Geometry check sheet. Reference: drawing and pictorial views, mm from the part's lowest x, y, z. Coordinates: 2 decimals unless noted, no trailing zeros. Write each loop counter-clockwise with the first axis right and the second up, starting at its lowest first coordinate (ties: lowest second). Pieces come first, ordered by that corner, then holes. Notation, with made-up numbers: (85, 26.25) -> (118, 26.25) arc R10 ccw to (118, 36.25) -> close; hole circle Ø10 at (37, -30). An arc over 180 degrees is marked (long way). Answer in a Markdown table with one row per item.
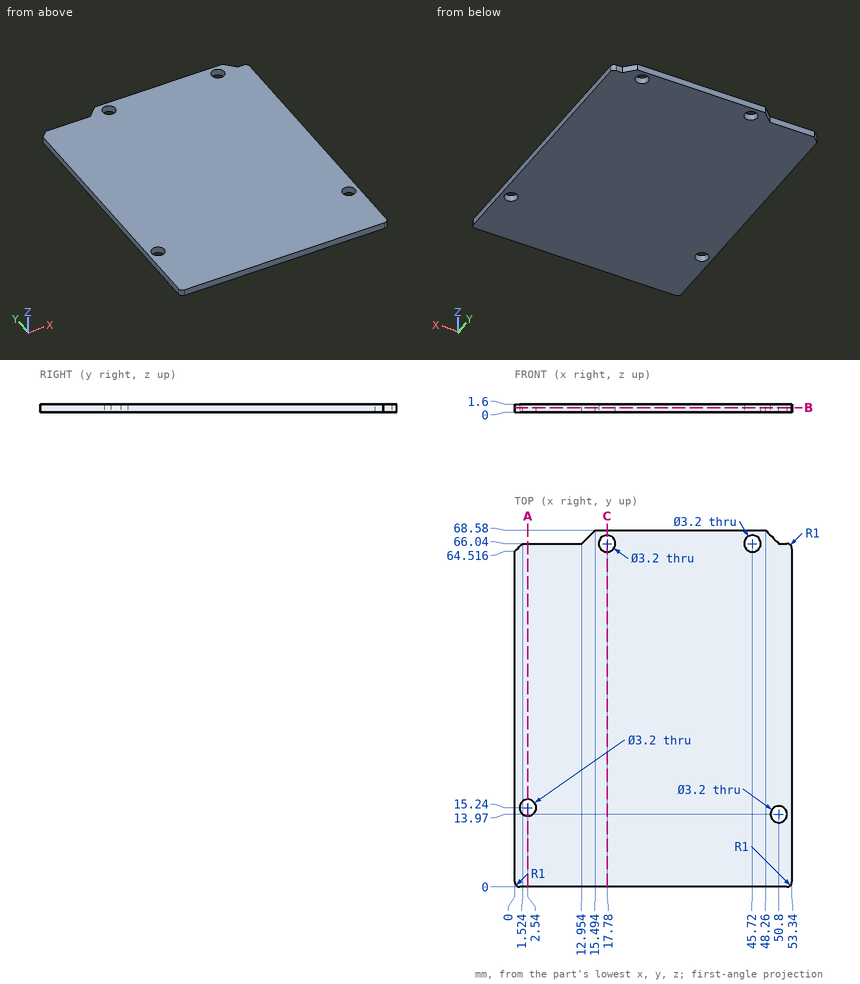
1. Thickness scan on line 1 (Y direction, x = 45.72, z = 1); line 2 (Y direction, x = 2.54, z = 0.6); line 3 (Y direction, x = 6, z = 0.5). Record the ranges inside material, lowest first. Write a range as from..to.
Geometry says:
| item | result |
|---|---|
| line 1 | 0..64.44, 67.64..68.58 |
| line 2 | 0..13.64, 16.84..66.04 |
| line 3 | 0..66.04 |
2. Section check C-C, the plane x = 17.78. Record the boundary of the cut face in (y, z).
Geometry says:
| item | result |
|---|---|
| outline | (0, 0) -> (64.44, 0) -> (64.44, 1.6) -> (0, 1.6) -> close; (67.64, 0) -> (68.58, 0) -> (68.58, 1.6) -> (67.64, 1.6) -> close |
3. Section check B-B, the plane z = 0.9. Record the boundary of the cut face in (x, y), plus the area to 3 significant figures.
Geometry says:
| item | result |
|---|---|
| outline | (0, 1) arc R1 ccw to (1, 0) -> (52.34, 0) arc R1 ccw to (53.34, 1) -> (53.34, 65.04) arc R1 ccw to (52.34, 66.04) -> (50.8, 66.04) -> (48.26, 68.58) -> (15.49, 68.58) -> (12.95, 66.04) -> (1.52, 66.04) -> (0, 64.52) -> close; hole circle Ø3.2 at (2.54, 15.24); hole circle Ø3.2 at (17.78, 66.04); hole circle Ø3.2 at (45.72, 66.04); hole circle Ø3.2 at (50.8, 13.97) |
| area | 3,580 mm^2 |
4. Section check A-A, the plane x = 2.54. Record the boundary of the cut face in (y, z).
Geometry says:
| item | result |
|---|---|
| outline | (0, 0) -> (13.64, 0) -> (13.64, 1.6) -> (0, 1.6) -> close; (16.84, 0) -> (66.04, 0) -> (66.04, 1.6) -> (16.84, 1.6) -> close |
5. Depth check by flat-ended pin: P1, Ø0.8, axis at x = 6, z = 0.5, coming from the +Y side; P2, Ø3.5, axis at x = 45.72, y = 66.04, coming from the +Z side. Enter the tip coordinate at first touch or a pass-through.
Geometry says:
| item | result |
|---|---|
| P1 | y = 66.04 |
| P2 | z = 1.6 |
